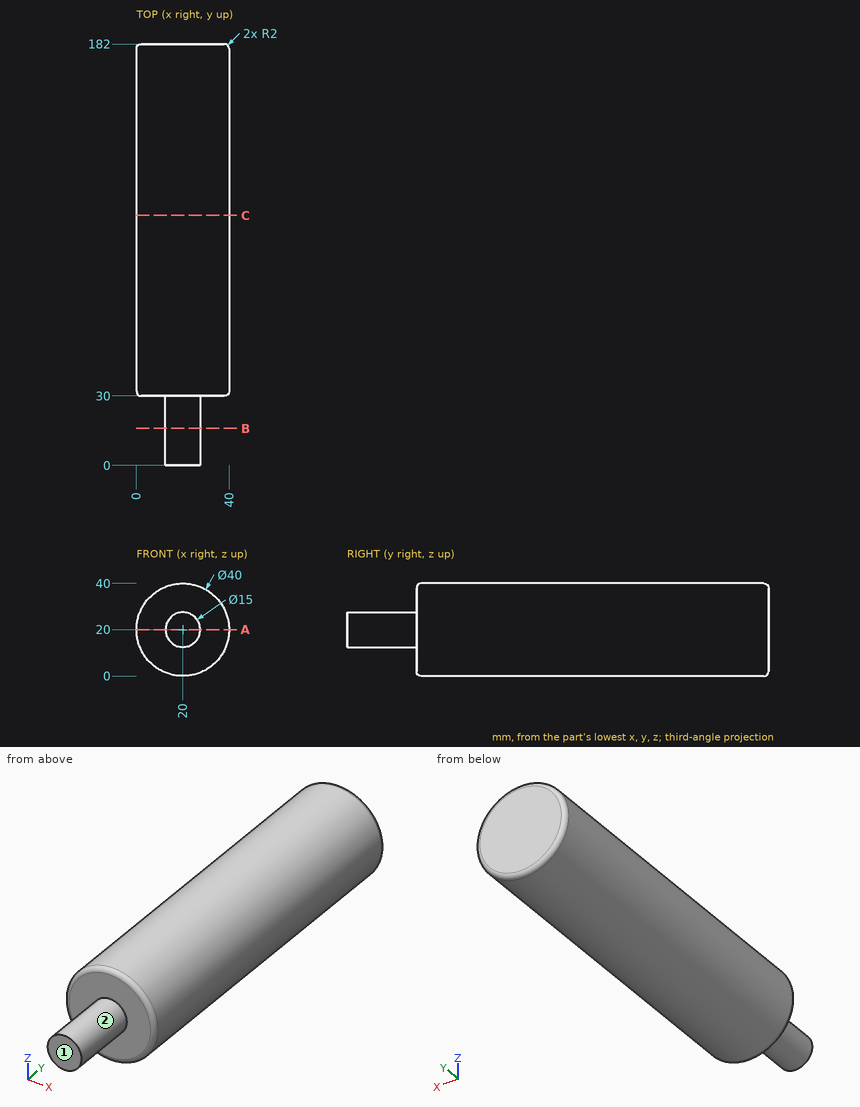
Part print with two shaded views. Sizes in mm from the minimum x, y, z corner. A direction names the side the tool comes from. Round coordinates to 2 decimals unless told otherwise and drop trailing zeros. Loops run counter-clockwise (first coordinate to the right, second up) from the corner with the lowest first, then second, coordinate; pieces in that order, holes last. Notation, with made-up numbers: M 80.25,27 L 139.25,27 A12 ccw 139.25,36 Z; hole C 35.25,11 d6. An arc over 180 degrees is marked long. Return JSON: item names as keys, results as strings. Group by question number.
(1) Wall check: probe 1 along Y at (x, z) = (32.5, 7.5); probe 2 along X at (y, z) = (100, 28.5); probe 3 along X at (y, z) = (140.5, 30). Give the ranges that are in metal, low to high. Write a range as [from, to].
(2) Tool access for the marked faces 1 and 2: list every direction of +Z, -Z, +X, -X, +Y, -Y with a clear straight run to the whole face (end or side of a thin tool).
(3) Saw through at C-C, the plane y = 108. List the corners of the cut face in (x, z).
(4) Drop flat-ended pins along their axis: P1, Ø1.5, axis at x = 33, y = 96.5, coming from the -Z side; P2, Ø2, axis at x = 12.5, y = 144.5, coming from the -Z side; P3, Ø1, axis at x = 14.5, y = 152.5, coming from the -Z side. Give the stop position or say it passes through.
(5) Saw through at B-B, the plane y = 16. List the corners of the cut face in (x, z), and give its area (3 significant figures).
(6) Saw through at A-A, the plane z = 20. List the corners of the cut face in (x, y), and give its area (3 significant figures).
Answer list:
{
 "1": {"probe 1": "[30, 182]", "probe 2": "[1.9, 38.1]", "probe 3": "[2.68, 37.32]"},
 "2": {"face 1": "+Z, -Z, +X, -X, -Y", "face 2": "-Y"},
 "3": {"outline": "C 20,20 d40"},
 "4": {"P1": "z = 4.19", "P2": "z = 1.09", "P3": "z = 0.64"},
 "5": {"outline": "C 20,20 d15", "area": "177 mm2"},
 "6": {"outline": "M 0,32 A2 ccw 2,30 L 12.5,30 L 12.5,0 L 27.5,0 L 27.5,30 L 38,30 A2 ccw 40,32 L 40,180 A2 ccw 38,182 L 2,182 A2 ccw 0,180 Z", "area": "6,530 mm2"}
}
